Autodesk Inventor part; units mm, degrees
ref_plane "YZ Plane" through (0, 0, 0) normal (1, 0, 0) x (0, 1, 0)
ref_plane "XZ Plane" through (0, 0, 0) normal (0, 1, 0) x (-1, 0, 0)
ref_plane "XY Plane" through (0, 0, 0) normal (0, 0, 1) x (1, 0, 0)
sketch "スケッチ1" plane through (0, 0, 0) normal (0, 0, 1) x (1, 0, 0)
  line L0 (-50, 0) -> (50, 0) construction
  circle A0 centre (-50, 0) radius 4
  circle A1 centre (50, 0) radius 6
  line L1 (-50, 11.35) -> (-23, 11.35)
  line L2 (-50, -11.35) -> (50, -11.35)
  arc A2 (50, -11.35) -> (50, 11.35) centre (50, 0) ccw
  line L3 (30, 25) -> (-15, 25)
  line L4 (-15, 25) -> (-23, 11.35)
  line L5 (-19.1026, 18) -> (41.8474, 18) construction
  line L6 (-15, 25) -> (-15, 18) construction
  line L7 (30, 25) -> (30, 18) construction
  circle A3 centre (27.5, 21.5) radius 1.55
  circle A4 centre (-12.5, 21.5) radius 1.55
  circle A5 centre (7.5, 21.5) radius 1.55
  line L8 (-15, 21.5) -> (30, 21.5) construction
  line L9 (30, 24) -> (-15, 24) construction
  line L10 (-15, 24) -> (-15, 19) construction
  line L11 (-15, 19) -> (30, 19) construction
  line L12 (30, 19) -> (30, 24) construction
  line L13 (-23, 11.35) -> (50, 11.35)
  arc A6 (-50, 11.35) -> (-50, -11.35) centre (-50, 0) ccw
  line L14 (7.5, 25) -> (7.5, 18.5172) construction
  line L15 (30, 25) -> (55.7736, 9.7718)
  point P0 (0, 0)
  point P1 (0, 0)
  point P2 (55.7736, 9.7718)
  point P3 (38, 11.35)
  dimension "d0" = 100
  dimension "d1" = 8
  dimension "d8" = 12
  dimension "d10" = 7
  dimension "d11" = 45
  dimension "d12" = 2.5
  dimension "d13" = 3.1
  dimension "d14" = 2.5
  dimension "d15" = 20
  dimension "d17" = 5
  dimension "d18" = 19
  dimension "d69" = 11.35
  dimension "d72" = 11.35
  dimension "d87" = 8
  dimension "d88" = 8
extrude "押し出し1" add sketch "スケッチ1" along normal blind 2
fillet "フィレット1" radius 5 4 edges at (-23, 11.35, 1) (-15, 25, 1) (30, 25, 1) (-50, 11.35, 1)
sketch "スケッチ2" plane through (0, 0, 2) normal (0, 0, 1) x (1, 0, 0)
  arc A0 (50, -11.35) -> (55.7736, 9.7718) centre (50, 0) ccw
  line L0 (18, -20) -> (-35.4549, -20) construction
  line L1 (-76.9372, -11.5) -> (-72, -11.5)
  line L2 (-76.9372, -12.4) -> (-76.9372, -11.5)
  line L3 (-71.9872, -11.45) -> (-76.9872, -11.45)
  line L4 (-76.9872, -11.45) -> (-76.9872, -12.45)
  circle A1 centre (-50, 0) radius 4
  circle A2 centre (-50, 0) radius 5.5 construction
  circle A3 centre (50, 0) radius 6
  line L5 (83.3205, -17.7128) -> (50, 0) construction
  line L6 (50, 0) -> (18, -20) construction
  line L7 (83.3205, -17.7128) -> (37.8533, -17.7128) construction
  line L8 (-13.4166, -12.4128) -> (46.4577, -12.4128)
  line L9 (46.4577, -12.4128) -> (46.4577, -11.5128)
  line L10 (46.4577, -11.5128) -> (45.5205, -11.5128)
  line L11 (45.5205, -11.5128) -> (35.5205, -7.0128)
  line L12 (35.5205, -7.0128) -> (-2.4795, -7.0128)
  line L13 (-2.4795, -7.0128) -> (-12.4795, -11.5128)
  line L14 (-12.4795, -11.5128) -> (-13.4166, -11.5128)
  line L15 (-13.4166, -11.5128) -> (-13.4166, -12.4128)
  line L16 (-12.4902, -11.4628) -> (-2.4902, -6.9628)
  line L17 (-2.4902, -6.9628) -> (35.5312, -6.9628)
  line L18 (35.5312, -6.9628) -> (45.5312, -11.4628)
  line L19 (45.5312, -11.4628) -> (46.5077, -11.4628)
  line L20 (46.5077, -11.4628) -> (46.5077, -12.4628)
  line L21 (46.5077, -12.4628) -> (-13.4666, -12.4628)
  line L22 (-13.4666, -12.4628) -> (-13.4666, -11.4628)
  line L23 (-13.4666, -11.4628) -> (-12.4902, -11.4628)
  point P0 (56.6914, 9.1677)
  point P1 (0, 0)
  point P2 (50, 11.35)
  dimension "d19" = 20
  dimension "d20" = 32
  dimension "d32" = 11
  dimension "d33" = 120
  dimension "d37" = 37.8
  dimension "d38" = 6.2
  dimension "d39" = 0.05
  dimension "d49" = 38
  dimension "d50" = 10
  dimension "d51" = 10
  dimension "d52" = 4.5
  dimension "d53" = 0.9
  dimension "d54" = 59.9743
extrude "押し出し2" cut sketch "スケッチ2" against normal blind 10 contours L15 L14 L13 L12 L11 L10 L9 L8 | L16 L17 L18 L19 L20 L21 L22 L23
fillet "フィレット2" radius 2 4 edges at (45.2805, -11.35, 1) (-12.2395, -11.35, 1) (35.5312, -6.9628, 1) (-2.4902, -6.9628, 1)
sketch "スケッチ4" plane through (0, 0, 2) normal (0, 0, 1) x (1, 0, 0)
  circle A0 centre (50, 0) radius 6
  circle A1 centre (50, 0) radius 8.5 construction
  line L0 (50, 0) -> (50, 8.5) construction
  circle A2 centre (50, 8.5) radius 1.35
  circle A3 centre (41.5, 0) radius 1.35
  circle A4 centre (50, -8.5) radius 1.35
  circle A5 centre (58.5, 0) radius 1.35
  point P0 (0, 0)
  dimension "d61" = 17
  dimension "d62" = 2.7
  dimension "d65" = 360
extrude "押し出し4" cut sketch "スケッチ4" against normal through all contours A2 | A3 | A4 | A5
sketch "スケッチ6" plane through (0, 0, 2) normal (0, 0, 1) x (1, 0, 0)
  circle A0 centre (-50, 0) radius 4
  circle A1 centre (-50, 0) radius 8.5 construction
  circle A2 centre (-58.5, 0) radius 2.5
  line L0 (-50, 0) -> (-58.5, 0) construction
  line L1 (-50, 0) -> (-41.5, 0) construction
  circle A3 centre (-41.5, 0) radius 2.5
  arc A4 (-50, 11.35) -> (-50, -11.35) centre (-50, 0) ccw
  line L2 (-58.5, -2.5) -> (-61.0712, -2.5)
  line L3 (-58.5, 2.5) -> (-61.0712, 2.5)
  point P0 (0, 0)
  dimension "d78" = 17
  dimension "d79" = 5
  dimension "d82" = 360
extrude "押し出し6" cut sketch "スケッチ6" against normal through all contours A2 | A2 L2 A4 L3 | A3
fillet "フィレット4" radius 2 2 edges at (-61.0712, 2.5, 1) (-61.0712, -2.5, 1)
equation "\"d14\" = d12"
properties part number "Link_front_side_frame" material "GFRP"
Design review of the part built by this model. Coordinates are the model's own, in mm. A direction names the side the tool comes from. Give positions to 0.01 mm unless a question says otherwise; leave off trailing zeros. Order: outer loops, then holes, each group sorted by start corner. A loop starts at its lowest first (then second) coordinate and runs counter-clockwise, first axis right, second up. Notation, with made-up numbers: (-18.75, 48) -> (-12.75, 48) arc R11 ccw to (-12.75, 55) -> close; hole circle Ø10 at (65, -12). An arc over 180 degrees is marked (long way). Write item = value, one per line. Start each with the question number.
(1) To check wall thickness, follow line 1 along Y through (x, z) = (-41.5, 0.8); line 2 along Y through (x, z) = (7.5, 1.15); line 3 along X through (y, z) = (-1, 1.3). State the ranges of each line that lie inside material, in increasing order.
(2) Mouldability with a two-part tool opening along X and no side actions: class faces 4 (the face through (7.298, 19.963, 0.986)), 5 (the face through (-32, -11.35, 1)), 6 (the face through (-18.96, 18.24, 0.99)), 7 (the face through (44, 0, 1)) as +X half, -X half, draft (parallel to the pull), parting line (faces both ways), or undercut.
(3) We need section D-D on y = -8.5. Write out the cut boundary in (x, z).
(4) We need section C-C on z = 0.65. State how many separate pieces and enclosed holes the cut face has, plus the area to 3 significant figures.
(5) We need section B-B on y = 8.5. Write out the cut boundary in (x, z).
(6) For faces 1 (the face through (-39.19, -0.96, 1.01)), 2 (the face through (-7.428, -9.185, 1.014)), 3 (the face through (-38, 11.35, 1)), list the 3-axis set-ups (+Z, -Z, +X, -X, +Y, -Y) from which the entire face can be reached by the end or side of a thin tool; tool diameter is ignored.
(7) For pin 1 (0.6 mm diameter, centred on x = -34, z = 1, fed in from +Y); pin 2 (1 mm diameter, centred on x = 22.5, z = 1, fed in from -Y), all flat-tipped, find the tip position at first contact; note any pin that passes through.
(8) We need section A-A on x = -41.5. Write out the cut boundary in (y, z), plus the area to 3 significant figures.
Numbers:
q1.line_1 = -11.35 to -2.5, 2.5 to 11.35
q1.line_2 = -6.96 to 19.95, 23.05 to 25
q1.line_3 = -56.21 to -53.87, -46.13 to -43.79, -39.21 to 40.59, 42.41 to 44.08, 55.92 to 57.59, 59.41 to 61.31
q2.face_4 = undercut
q2.face_5 = draft
q2.face_6 = -X half
q2.face_7 = undercut
q3.outline = (-57.52, 0) -> (-5.91, 0) -> (-5.91, 2) -> (-57.52, 2) -> close; (38.95, 0) -> (48.65, 0) -> (48.65, 2) -> (38.95, 2) -> close; (51.35, 0) -> (57.52, 0) -> (57.52, 2) -> (51.35, 2) -> close
q4.separate_pieces = 1
q4.enclosed_holes = 10
q4.area = 3,040 mm^2
q5.outline = (-57.52, 0) -> (48.65, 0) -> (48.65, 2) -> (-57.52, 2) -> close; (51.35, 0) -> (57.52, 0) -> (57.52, 2) -> (51.35, 2) -> close
q6.face_1 = +Z, -Z
q6.face_2 = +Z, -Z, -Y
q6.face_3 = +Z, -Z, -X, +Y
q7.pin_1 = 11.35
q7.pin_2 = -6.96
q8.outline = (-11.35, 0) -> (-2.5, 0) -> (-2.5, 2) -> (-11.35, 2) -> close; (2.5, 0) -> (11.35, 0) -> (11.35, 2) -> (2.5, 2) -> close
q8.area = 35.4 mm^2
